Build history of the part. All positions in model axes, mm. A direction names the side the tool comes from. Coordinates: 2 decimals unless noted, no trailing zeros. Write each loop counter-clockwise with the first axis right and the second up, starting at its lowest first coordinate (ties: lowest second). Pieces come first, ordered by that corner, then holes.
from build123d import *

# Parameters (mm, degrees)
SKETCH_1_W        = 21.7
SKETCH_1_H        = 21.7
SKETCH_1_R        = 1
SKETCH_1_R_2      = 7
EXTRUDE_1_DEPTH   = 1.4
SKETCH_2_R        = 7
SKETCH_2_R_2      = 6.5
EXTRUDE_1_2_DEPTH = 12.7


with BuildPart() as part:
    # Эскиз1 → Extrude 1 (new body)
    with BuildSketch(Plane.XY):
        with Locations((10.85, 10.85)):
            Rectangle(SKETCH_1_W, SKETCH_1_H)
        with Locations((2.6, 19.1)):
            Circle(SKETCH_1_R, mode=Mode.SUBTRACT)
        with Locations((10.85, 10.85)):
            Circle(SKETCH_1_R_2, mode=Mode.SUBTRACT)
        with Locations((19.1, 19.1)):
            Circle(SKETCH_1_R, mode=Mode.SUBTRACT)
        with Locations((19.1, 2.6)):
            Circle(SKETCH_1_R, mode=Mode.SUBTRACT)
        with Locations((2.6, 2.6)):
            Circle(SKETCH_1_R, mode=Mode.SUBTRACT)
    extrude(amount=EXTRUDE_1_DEPTH)

    # Эскиз2 → Extrude 1 2 (add)
    with BuildSketch(Plane(origin=(0, 0, 0), x_dir=(-1, 0, 0), z_dir=(0, 0, -1))):
        with Locations((-10.85, 10.85)):
            Circle(SKETCH_2_R)
        with Locations((-10.85, 10.85)):
            Circle(SKETCH_2_R_2, mode=Mode.SUBTRACT)
    extrude(amount=-EXTRUDE_1_2_DEPTH)


solid = part.part
(1) Slice it at D-D, the plane x = 18.5. List the corners of the cut face in (y, z), and give its area (3 significant figures).
(2) Slice it at C-C, the plane y = 19.1. List the corners of the cut face in (x, z).
(3) Two-plate mould, pull along X, no slides. Class faces 3 (the flat face through (21.7, 11, 1)), 4 (the cylindrical face through (19.56, 18.21, 0.69)), 5 (the flat face through (11, 0, 1)), 6 (the cylindrical face through (15.641, 15.243, 6.261)): pulls with the +X half, pulls with the -X half, needs draft (parallel to the pull), parting line crosses it, or undercut.
(4) Slice it at A-A, the plane y = 10.85. List the corners of the cut face in (x, z), and give its area (3 significant figures).
(5) Flat gauge pins, fed straight in: P1, Ø6, axis at x = 12.5, z = 5.5, coming from the -Y side; P2, Ø12, axis at x = 6, y = 17.5, coming from the -Z side; P3, Ø3, axis at y = 7, z = 4.5, coming from the +X side; P4, Ø2.5, axis at x = 2.6, y = 2.6, coming from the +Z side. Where does each tip first touch, or does it go through?
(6) Probe L1, parallel to Y at x = 19.1, z = 1; L2, parallel to Y at x = 10.85, z = 7.5; L3, parallel to Z at x = 2.75, y = 10. List the from-to ranges inside material, lowest first.
(7) 3-axis set-ups, long thin cutter, end or side, ignore diameter. For faces 1 (the flat face through (11, 18, 1.4)), 2 (the cylindrical face through (3.554, 2.9, 0.69)): which of +Z, -Z, +X, -X, +Y, -Y reach the whole face in a straight line?
Results:
1. outline: (0, 0) - (1.8, 0) - (1.8, 1.4) - (0, 1.4) - close; (3.4, 0) - (18.3, 0) - (18.3, 1.4) - (3.4, 1.4) - close; (19.9, 0) - (21.7, 0) - (21.7, 1.4) - (19.9, 1.4) - close
1. area: 25.9 mm2
2. outline: (0, 0) - (1.6, 0) - (1.6, 1.4) - (0, 1.4) - close; (3.6, 0) - (18.1, 0) - (18.1, 1.4) - (3.6, 1.4) - close; (20.1, 0) - (21.7, 0) - (21.7, 1.4) - (20.1, 1.4) - close
3. face 3: pulls with the +X half
3. face 4: undercut
3. face 5: needs draft
3. face 6: undercut
4. outline: (0, 0) - (4.35, 0) - (4.35, 12.7) - (3.85, 12.7) - (3.85, 1.4) - (0, 1.4) - close; (17.35, 0) - (21.7, 0) - (21.7, 1.4) - (17.85, 1.4) - (17.85, 12.7) - (17.35, 12.7) - close
4. area: 23.5 mm2
5. P1: stops at y = 3.85
5. P2: stops at z = 0
5. P3: stops at x = 17.44
5. P4: stops at z = 1.4
6. L1: y = 0 to 1.6, 3.6 to 18.1, 20.1 to 21.7
6. L2: y = 3.85 to 4.35, 17.35 to 17.85
6. L3: z = 0 to 1.4
7. face 1: +Z
7. face 2: +Z, -Z
